from build123d import *

# Parameters (mm, degrees)
BOSS_EXTRUDE2_DEPTH      = 22.5
BOSS_EXTRUDE2_DEPTH_BACK = 22.5
SKETCH4_W                = 45
SKETCH4_H                = 45
CUT_EXTRUDE1_DEPTH       = 22.5
CUT_EXTRUDE1_DEPTH_BACK  = 20.5
SKETCH5_W                = 41
SKETCH5_H                = 41
SKETCH6_R                = 1.5
CUT_EXTRUDE2_DEPTH       = 32.5
SKETCH8_R                = 1
CUT_EXTRUDE3_DEPTH       = 32.5
SKETCH9_W                = 7.5
SKETCH9_H                = 3.5
CUT_EXTRUDE4_DEPTH       = 32.5
FILLET2_R                = 1
FILLET3_R                = 2


with BuildPart() as part:
    # Sketch4 → Boss-Extrude2 (new, two sides: drawn at the far end of the back side and taken through both)
    with BuildSketch(Plane(origin=(0, 0, 0), x_dir=(1, 0, 0), z_dir=(0, 1, 0)).offset(-BOSS_EXTRUDE2_DEPTH_BACK)):
        Rectangle(SKETCH4_W, SKETCH4_H)
    extrude(amount=BOSS_EXTRUDE2_DEPTH + BOSS_EXTRUDE2_DEPTH_BACK)

    # Sketch5 → Cut-Extrude1 (cut, two sides: drawn at the far end of the back side and taken through both)
    with BuildSketch(Plane(origin=(0, 0, 0), x_dir=(1, 0, 0), z_dir=(0, 1, 0)).offset(-CUT_EXTRUDE1_DEPTH_BACK)):
        Rectangle(SKETCH5_W, SKETCH5_H)
    extrude(amount=CUT_EXTRUDE1_DEPTH + CUT_EXTRUDE1_DEPTH_BACK, mode=Mode.SUBTRACT)

    # Sketch6 → Cut-Extrude2 (cut)
    with BuildSketch(Plane.XY):
        with Locations(Location((2, 10, 0), (0, 0, 180))):
            Circle(SKETCH6_R)
        with Locations(Location((6, 10, 0), (0, 0, 180))):
            Circle(SKETCH6_R)
        with Locations(Location((-2, 10, 0), (0, 0, 180))):
            Circle(SKETCH6_R)
        with Locations(Location((-6, 10, 0), (0, 0, 180))):
            Circle(SKETCH6_R)
    extrude(amount=CUT_EXTRUDE2_DEPTH, mode=Mode.SUBTRACT)

    # Sketch8 → Cut-Extrude3 (cut)
    with BuildSketch(Plane.XY):
        Circle(SKETCH8_R)
        with Locations((3, 0)):
            Circle(SKETCH8_R)
        with Locations((0, 3)):
            Circle(SKETCH8_R)
        with Locations((-3, 0)):
            Circle(SKETCH8_R)
        with Locations((0, -3)):
            Circle(SKETCH8_R)
    extrude(amount=-CUT_EXTRUDE3_DEPTH, mode=Mode.SUBTRACT)

    # Sketch9 → Cut-Extrude4 (cut)
    with BuildSketch(Plane.XY):
        with Locations((0, -14.75)):
            Rectangle(SKETCH9_W, SKETCH9_H)
    extrude(amount=-CUT_EXTRUDE4_DEPTH, mode=Mode.SUBTRACT)

    # Fillet2
    fillet2_edges = [part.edges().sort_by_distance(p)[0] for p in [
        (-3.75, -16.5, -21.5),
        (-3.75, -13, -21.5),
        (3.75, -13, -21.5),
        (3.75, -16.5, -21.5),
    ]]
    fillet(fillet2_edges, radius=FILLET2_R)

    # Fillet3
    fillet3_edges = [part.edges().sort_by_distance(p)[0] for p in [
        (-22.5, 0, -22.5),
        (22.5, 0, -22.5),
        (22.5, 0, 22.5),
        (-22.5, 0, 22.5),
    ]]
    fillet(fillet3_edges, radius=FILLET3_R)


solid = part.part
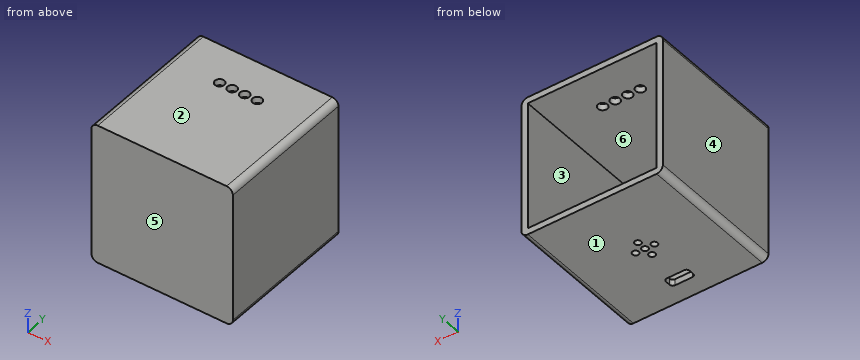
Here's how the part is built. I have some questions about the finished solid (model axes, mm). Face numbers are marked on the shaded views. A direction names the side the tool comes from. Round coordinates to 2 decimals unless told otherwise and drop trailing zeros. Loops run counter-clockwise (first coordinate to the right, second up) from the corner with the lowest first, then second, coordinate; pieces in that order, holes last. Notation, with made-up numbers: M -37,-1.75 L -33,-1.75 A31 ccw -33,28.25 Z; hole C 26,12.5 d5. An arc over 180 degrees is marked long. Write each question's results on one line, items separated by ' | '. Start each with the question number.
(1) If I drill on probe 1 along Z at (x, y) = (14.5, -5); probe 2 along Y at (x, z) = (-2, 21.5), over which ranges is the centre line in solid material (lowest first)? Write a range as from..to.
(2) I want a section at D-D (z = 11). Please give me the cut outline in (x, y).
(3) On a 3-axis mill with a long thin cutter (end or side, diameter ignored), from which of +Z, -Z, +X, -X, +Y, -Y can I reach the whole of each face in a straight line? I mean the marked faces 5 and 6. Say none if no direction works.
(4) I want a section at B-B (y = -3). Please give me the cut outline in (x, z), then the cut area to 3 significant figures.
(5) I want a section at C-C (x = -12.5). Please give me the cut outline in (y, z), then the cut area to 3 significant figures.
(6) Thinking about a two-plate mould opening in Z: for the marked faces 1, 2, 3 and 4, which applies, pulls with the +Z half, pulls with the -Z half, needs draft (parallel to the pull), parting line crosses it, or undercut?
(7) Will these pins go through, and if not, where does the flat tip stop? P1, Ø1.6, axis at y = -15, z = -21.5, coming from the -X side; P2, Ø1.2, axis at y = -14.5, z = -22, coming from the +X side; P3, Ø12, axis at x = -5.5, z = 10.5, coming from the +Y side; P4, Ø12, axis at x = 7.5, z = 17, coming from the +Y side.
(8) I want a section at A-A (x = 6). Please give me the cut outline in (y, z), then the cut area to 3 significant figures.
Solved:
1) probe 1: z = -22.5..-20.5, 20.5..22.5 | probe 2: y = -22.5..8.5, 11.5..22.5
2) outline: M -22.5,-22.5 L 22.5,-22.5 L 22.5,22.5 L 20.5,22.5 L 20.5,-20.5 L -20.5,-20.5 L -20.5,22.5 L -22.5,22.5 Z
3) face 5: +Z, -Z, +X, -X, -Y | face 6: +Y
4) outline: M -22.5,-20.5 A2 ccw -20.5,-22.5 L -1,-22.5 L -1,-20.5 L -20.5,-20.5 L -20.5,20.5 L 20.5,20.5 L 20.5,-20.5 L 1,-20.5 L 1,-22.5 L 20.5,-22.5 A2 ccw 22.5,-20.5 L 22.5,20.5 A2 ccw 20.5,22.5 L -20.5,22.5 A2 ccw -22.5,20.5 Z | area: 337 mm²
5) outline: M -22.5,-22.5 L 22.5,-22.5 L 22.5,-20.5 L -20.5,-20.5 L -20.5,20.5 L 22.5,20.5 L 22.5,22.5 L -22.5,22.5 Z | area: 262 mm²
6) face 1: pulls with the -Z half | face 2: pulls with the +Z half | face 3: undercut | face 4: needs draft
7) P1: stops at x = -22.49 | P2: stops at x = 22.29 | P3: stops at y = -20.5 | P4: stops at y = 22.5
8) outline: M -22.5,-22.5 L 22.5,-22.5 L 22.5,-20.5 L -20.5,-20.5 L -20.5,20.5 L 8.5,20.5 L 8.5,22.5 L -22.5,22.5 Z; M 11.5,20.5 L 22.5,20.5 L 22.5,22.5 L 11.5,22.5 Z | area: 256 mm²
